CAD build for the part. Positions are in the model's coordinates, mm. Face numbers are marked on the shaded views. Give positions to 0.01 mm unless a question says otherwise; leave off trailing zeros. Write each loop counter-clockwise with the first axis right and the second up, starting at its lowest first coordinate (ties: lowest second). Pieces come first, ordered by that corner, then holes. Notation, with made-up numbers: (53.25, -22) -> (104.25, -22) arc R15 ccw to (104.25, 5) -> close; hole circle Ø6 at (38, 5.25). An arc over 180 degrees is marked (long way). Answer as a JSON object with one key per item and string values.
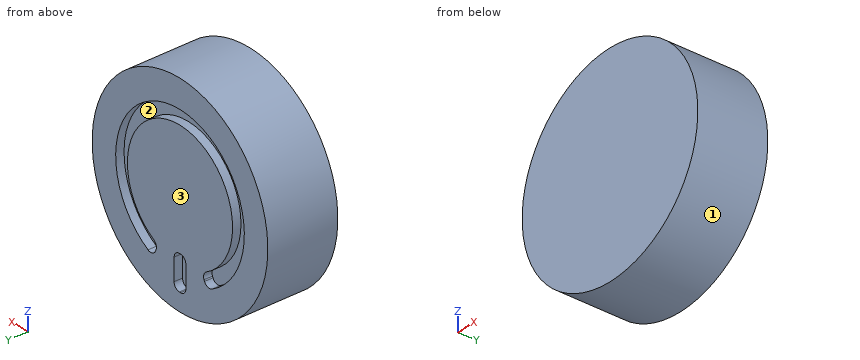
```python
from build123d import *

# Parameters (mm, degrees)
SKETCH1_R           = 14.95
BOSS_EXTRUDE1_DEPTH = 10
CUT_EXTRUDE1_DEPTH  = 1.2


with BuildPart() as part:
    # Sketch1 → Boss-Extrude1 (new body)
    with BuildSketch(Plane(origin=(0, 0, 0), x_dir=(1, 0, 0), z_dir=(0, 1, 0))):
        with Locations(Location((0, 0, 0), (0, 0, 270))):  # turned: the seam where the file's is
            Circle(SKETCH1_R)
    extrude(amount=BOSS_EXTRUDE1_DEPTH)

    # Sketch2 → Cut-Extrude1 (cut)
    with BuildSketch(Plane(origin=(0, 10, 0), x_dir=(1, 0, 0), z_dir=(0, 1, 0))):
        with BuildLine():
            ThreePointArc((1, 8.893958624), (0, 8.95), (-1, 8.893958624))
            Line((-1, 8.893958624), (-1, 8.379586094))
            ThreePointArc((-1, 8.379586094), (-0.736396103, 7.743189991), (-0.1, 7.479586094))
            Line((-0.1, 7.479586094), (0.1, 7.479586094))
            ThreePointArc((0.1, 7.479586094), (0.736396103, 7.743189991), (1, 8.379586094))
            Line((1, 8.379586094), (1, 8.893958624))
        make_face()
        with BuildLine():
            ThreePointArc((1, 10.904242294), (0, 10.95), (-1, 10.904242294))
            Line((-1, 10.904242294), (-1, 8.893958624))
            ThreePointArc((-1, 8.893958624), (0, 8.95), (1, 8.893958624))
            Line((1, 8.893958624), (1, 10.904242294))
        make_face()
        with BuildLine():
            Line((0.1, 12.420413906), (-0.1, 12.420413906))
            ThreePointArc((-0.1, 12.420413906), (-0.736396103, 12.156810009), (-1, 11.520413906))
            Line((-1, 11.520413906), (-1, 10.904242294))
            ThreePointArc((-1, 10.904242294), (0, 10.95), (1, 10.904242294))
            Line((1, 10.904242294), (1, 11.520413906))
            ThreePointArc((1, 11.520413906), (0.736396103, 12.156810009), (0.1, 12.420413906))
        make_face()
        with BuildLine():
            ThreePointArc((-4.464100977, 7.757209709), (0, -8.95), (4.464100977, 7.757209709))
            ThreePointArc((4.464100977, 7.757209709), (4.055618077, 8.263608167), (4.095196767, 8.913016517))
            Line((4.095196767, 8.913016517), (4.179040986, 9.09549979))
            ThreePointArc((4.179040986, 9.09549979), (4.722410459, 9.57688432), (5.444328238, 9.500620508))
            ThreePointArc((5.444328238, 9.500620508), (0, -10.95), (-5.444328238, 9.500620508))
            ThreePointArc((-5.444328238, 9.500620508), (-4.722410459, 9.57688432), (-4.179040986, 9.09549979))
            Line((-4.179040986, 9.09549979), (-4.095196767, 8.913016517))
            ThreePointArc((-4.095196767, 8.913016517), (-4.055618077, 8.263608167), (-4.464100977, 7.757209709))
        make_face()
    extrude(amount=-CUT_EXTRUDE1_DEPTH, mode=Mode.SUBTRACT)


solid = part.part
```
1) Pin check, flat tips, straight feed: pin 1 (3 mm diameter, centred on x = 5, y = 7, fed in from +Z); pin 2 (3 mm diameter, centred on x = -4.5, y = 4.5, fed in from -Z); pin 3 (3 mm diameter, centred on x = 7, y = 7.5, fed in from +Z). Stop position of each tip, or through.
Model answer:
{"pin 1": "stops at z = 14.53", "pin 2": "stops at z = -14.65", "pin 3": "stops at z = 13.9"}
2) Slice it at C-C (y = 5). List the corners of the cut face in (x, z).
Model answer:
{"outline": "circle Ø29.9 at (0, 0)"}
3) Wall check: probe 1 along X at (y, z) = (9.75, 0); probe 2 along Y at (x, z) = (10.25, 2.5); probe 3 along Z at (x, y) = (0.25, 3.5). Give the ranges that are in metal, low to high.
Model answer:
{"probe 1": "x = -14.95 to -10.95, -8.95 to 8.95, 10.95 to 14.95", "probe 2": "y = 0 to 8.8", "probe 3": "z = -14.95 to 14.95"}
4) Slice it at A-A (z = 0). List the corners of the cut face in (x, y), then the cut area to 3 significant figures.
Model answer:
{"outline": "(-14.95, 0) -> (14.95, 0) -> (14.95, 10) -> (10.95, 10) -> (10.95, 8.8) -> (8.95, 8.8) -> (8.95, 10) -> (-8.95, 10) -> (-8.95, 8.8) -> (-10.95, 8.8) -> (-10.95, 10) -> (-14.95, 10) -> close", "area": "294 mm2"}
5) Mould opens along Z. For the marked faces 1, 2 and 3 say: released by +Z, released by -Z, zero draft, split by the parting line, or undercut.
Model answer:
{"face 1": "split by the parting line", "face 2": "undercut", "face 3": "zero draft"}
6) Slice it at D-D (z = -6). List the corners of the cut face in (x, y).
Model answer:
{"outline": "(-13.69, 0) -> (13.69, 0) -> (13.69, 10) -> (9.16, 10) -> (9.16, 8.8) -> (6.64, 8.8) -> (6.64, 10) -> (-6.64, 10) -> (-6.64, 8.8) -> (-9.16, 8.8) -> (-9.16, 10) -> (-13.69, 10) -> close"}
7) Slice it at B-B (x = -3). List the corners of the cut face in (y, z), then the cut area to 3 significant figures.
Model answer:
{"outline": "(0, -14.65) -> (10, -14.65) -> (10, 8.43) -> (8.8, 8.43) -> (8.8, 10.53) -> (10, 10.53) -> (10, 14.65) -> (0, 14.65) -> close", "area": "290 mm2"}
